Model file for the job. Use its own axes, mm. A direction names the side the tool comes from. Coordinates: 2 decimals unless noted, no trailing zeros. Order: outer loops, then holes, each group sorted by start corner. A loop starts at its lowest first (then second) coordinate and runs counter-clockwise, first axis right, second up.
Autodesk Inventor part; units mm, degrees
ref_plane "YZ Plane" through (0, 0, 0) normal (1, 0, 0) x (0, 1, 0)
ref_plane "XZ Plane" through (0, 0, 0) normal (0, 1, 0) x (-1, 0, 0)
ref_plane "XY Plane" through (0, 0, 0) normal (0, 0, 1) x (1, 0, 0)
sketch "Sketch1" plane through (0, 0, 0) normal (0, 1, 0) x (-1, 0, 0)
  line L0 (-13.3, 9.8) -> (13.3, 9.8)
  line L1 (13.3, 9.8) -> (13.3, -9.8)
  line L2 (13.3, -9.8) -> (-13.3, -9.8)
  line L3 (-13.3, -9.8) -> (-13.3, 9.8)
  line L4 (-13.3, 9.8) -> (13.3, -9.8) construction
  line L5 (13.3, 9.8) -> (-13.3, -9.8) construction
  point P0 (0, 0)
  dimension "d0" = 26.6
  dimension "d1" = 19.6
extrude "Extrusion1" add sketch "Sketch1" along normal blind 2
sketch "Sketch2" plane through (0, 0, 0) normal (0, -1, 0) x (1, 0, 0)
  line L0 (13.3, 9.8) -> (-13.3, 9.8)
  line L1 (13.3, -9.8) -> (13.3, 9.8)
  line L2 (-14.3, -10.8) -> (14.3, -10.8)
  line L3 (14.3, -10.8) -> (14.3, 10.8)
  line L4 (14.3, 10.8) -> (-14.3, 10.8)
  line L5 (-14.3, 10.8) -> (-14.3, -10.8)
  line L6 (-14.3, -10.8) -> (14.3, 10.8) construction
  line L7 (14.3, -10.8) -> (-14.3, 10.8) construction
  point P0 (0, 0)
  dimension "d4" = 1
  dimension "d5" = 1
extrude "Extrusion2" add sketch "Sketch2" along normal blind 1
chamfer "Chamfer1" distance 1 angle 45 4 edges at (0, 0, 10.8) (-14.3, 0, 0) (14.3, 0, 0) (0, 0, -10.8)
sketch "Sketch3" plane through (0, -1, 0) normal (0, -1, 0) x (1, 0, 0)
  line L0 (14.3, -10.8) -> (14.3, 10.8)
  line L1 (14.3, 10.8) -> (-14.3, 10.8)
  line L2 (-12.8, -9.3) -> (12.8, -9.3)
  line L3 (12.8, -9.3) -> (12.8, 9.3)
  line L4 (12.8, 9.3) -> (-12.8, 9.3)
  line L5 (-12.8, 9.3) -> (-12.8, -9.3)
  line L6 (-12.8, -9.3) -> (12.8, 9.3) construction
  line L7 (12.8, -9.3) -> (-12.8, 9.3) construction
  point P0 (0, 0)
  dimension "d11" = 1.5
  dimension "d12" = 1.5
extrude "Extrusion3" cut sketch "Sketch3" against normal blind 1
properties part number "wysw trans v2"
Q1. Mould opens along Z. For faces 1 (the face through (-0.2, -0.5, -9.3)), 2 (the face through (0, 2, 0)), 3 (the face through (0, 1, -9.8)) say: pulls with the +Z half, pulls with the -Z half, needs draft (parallel to the pull), parting line crosses it, or undercut.
Established:
face 1: undercut
face 2: needs draft
face 3: pulls with the -Z half
Q2. Cut at C-C, the plane y = -0.55. List the corners of the cut face in (x, z).
Established:
outline: (-13.85, -10.35) - (13.85, -10.35) - (13.85, 10.35) - (-13.85, 10.35) - close; hole (-12.8, -9.3) - (12.8, -9.3) - (12.8, 9.3) - (-12.8, 9.3) - close
Q3. Which spindle directions (+Z, -Z, +X, -X, +Y, -Y) get a long thin tool onto all of the face, cutting with end or side? Do faces 4 (the face through (0, 1, 9.8)), 5 (the face through (-13.3, 1, 0)), 6 (the face through (12.8, -0.5, -0.1)). Say none if no direction does.
Established:
face 4: +Z, +X, -X, +Y
face 5: +Z, -Z, -X, +Y
face 6: -Y
Q4. Probe line 1 (X direction, y = 1.25, z = 0.75); line 2 (Y direction, x = 12.75, z = 5.5); line 3 (Z direction, x = -11.75, y = 1.4). List the from-to ranges inside material, lowest first.
Established:
line 1: x = -13.3 to 13.3
line 2: y = 0 to 2
line 3: z = -9.8 to 9.8
Q5. Drop flat-ended pins along their axis: P1, Ø1.5, axis at y = 1.5, z = -8.5, coming from the -X side; P2, Ø0.8, axis at y = -0.5, z = 1, coming from the -X side; P3, Ø0.8, axis at y = -0.5, z = 1, coming from the +X side. Give the stop position or say it passes through.
Established:
P1: stops at x = -13.3
P2: stops at x = -14.2
P3: stops at x = 14.2
